Autodesk Inventor part; units mm, degrees
ref_plane "YZ Plane" through (0, 0, 0) normal (1, 0, 0) x (0, 1, 0)
ref_plane "XZ Plane" through (0, 0, 0) normal (0, 1, 0) x (-1, 0, 0)
ref_plane "XY Plane" through (0, 0, 0) normal (0, 0, 1) x (1, 0, 0)
sketch "Sketch1" plane through (0, 0, 0) normal (0, 0, 1) x (1, 0, 0)
  line L0 (0, 0) -> (140, 0)
  line L1 (140, 0) -> (140, 232.6)
  line L2 (140, 232.6) -> (90, 232.6)
  line L3 (90, 232.6) -> (90, 100)
  line L4 (90, 100) -> (50, 100)
  line L5 (50, 100) -> (50, 232.6)
  line L6 (50, 232.6) -> (0, 232.6)
  line L7 (0, 232.6) -> (0, 0)
  line L8 (30, 232.6) -> (30, 0) construction
  line L9 (70, 100) -> (70, 0) construction
  circle A0 centre (30, 192.6) radius 14 construction
  circle A1 centre (30, 152.6) radius 14 construction
  dimension "d3" = 40
  dimension "d6" = 28
  dimension "d7" = 40
  dimension "d8" = 40
  dimension "d9" = 132.6
  dimension "d10" = 100
  dimension "d36" = 20
  dimension "d37" = 50
extrude "Extrusion1" add sketch "Sketch1" along normal blind 3
ref_plane "Work Plane1" through (115, 0, 0) normal (1, 0, 0) x (0, 0, -1)
sketch "Sketch2" plane through (0, 0, 3) normal (0, 0, 1) x (1, 0, 0)
  line L0 (50, 232.6) -> (0, 232.6) construction
  line L1 (30, 232.6) -> (30, 50) construction
  line L2 (90, 100) -> (50, 100) construction
  line L3 (70, 100) -> (70, 0) construction
  line L4 (0, 0) -> (140, 0) construction
  circle A0 centre (30, 194.6) radius 14.25
  circle A1 centre (30, 134.6) radius 14.25
  circle A2 centre (30, 202.6) radius 4.6 construction
  circle A3 centre (110, 194.6) radius 14.25
  circle A4 centre (110, 134.6) radius 14.25
  line L5 (50, 100) -> (50, 232.6)
  dimension "d13" = 28.5
  dimension "d14" = 9.2
  dimension "d15" = 8
  dimension "d16" = 60
  dimension "d33" = 30
  dimension "d38" = 20
extrude "Extrusion2" cut sketch "Sketch2" against normal blind 10
sketch "Sketch3" plane through (0, 0, 3) normal (0, 0, 1) x (1, 0, 0)
  line L0 (5, 227.6) -> (45, 227.6)
  line L1 (45, 227.6) -> (45, 224.6)
  line L2 (45, 224.6) -> (5, 224.6)
  line L3 (5, 224.6) -> (5, 227.6)
  line L4 (53, 95) -> (87, 95)
  line L5 (87, 95) -> (87, 92)
  line L6 (87, 92) -> (53, 92)
  line L7 (53, 92) -> (53, 95)
  line L8 (5, 8) -> (135, 8)
  line L9 (135, 8) -> (135, 5)
  line L10 (135, 5) -> (5, 5)
  line L11 (5, 5) -> (5, 8)
  circle A0 centre (110, 194.6) radius 14.25
  circle A1 centre (30, 134.6) radius 14.25
  circle A2 centre (110, 134.6) radius 14.25
  circle A3 centre (30, 194.6) radius 14.25
  line L12 (50, 100) -> (50, 232.6)
  line L13 (50, 232.6) -> (0, 232.6)
  line L14 (0, 232.6) -> (0, 0)
  line L15 (0, 0) -> (140, 0)
  line L16 (140, 0) -> (140, 232.6)
  line L17 (140, 232.6) -> (90, 232.6)
  line L18 (90, 232.6) -> (90, 100)
  line L19 (90, 100) -> (50, 100)
  line L20 (90, 100) -> (50, 100) construction
  line L21 (70, 100) -> (70, 0) construction
  line L22 (0, 0) -> (140, 0) construction
  line L23 (135, 227.6) -> (95, 227.6)
  line L24 (95, 227.6) -> (95, 224.6)
  line L25 (95, 224.6) -> (135, 224.6)
  line L26 (135, 224.6) -> (135, 227.6)
  dimension "d20" = 5
  dimension "d21" = 5
  dimension "d22" = 5
  dimension "d23" = 3
  dimension "d24" = 5
  dimension "d25" = 3
  dimension "d26" = 3
  dimension "d27" = 3
  dimension "d28" = 5
  dimension "d29" = 3
  dimension "d30" = 5
extrude "Extrusion3" cut sketch "Sketch3" against normal blind 10 contours L0 L1 L2 L3 | L4 L5 L6 L7 | L8 L9 L10 L11 | L26 L25 L24 L23
ref_plane "Work Plane2" through (70, 0, 0) normal (1, 0, 0) x (0, 0, -1)
equation "\"d3\" = 0.5 * marshdistance"
equation "\"d9\" = sidewallL"
equation "\"d10\" = Uthick"
equation "\"d36\" = 0.5 * Utip"
equation "\"d16\" = marshmarshD"
equation "\"d33\" = marshedgeD"
equation "\"d38\" = 0.5 * Utip"
equation "\"thick\" = 0.5"
equation "\"lrlr\" = 19"
equation "\"lrmid\" = 19.9"
equation "\"lrdepth\" = 3.3"
equation "\"mlr\" = 16.6"
equation "\"mmid\" = 24.7"
equation "\"mdepth\" = 4.5"
equation "\"lrltotal\" = 126.6"
equation "\"mltotal\" = 126.6"
equation "\"lrbetween\" = 52.1"
equation "\"mbetween\" = 49.5"
equation "\"toler\" = 1"
equation "\"tight\" = 0.08"
equation "\"stuckw\" = 6"
equation "\"sidewallL\" = 132.6"
equation "\"heaterH\" = 117.3"
equation "\"Uthick\" = 100"
equation "\"marshmarshD\" = 60"
equation "\"marshedgeD\" = 30"
equation "\"stickL\" = 3.5"
equation "\"wireH\" = 25"
properties part number "Ushape_bottom"
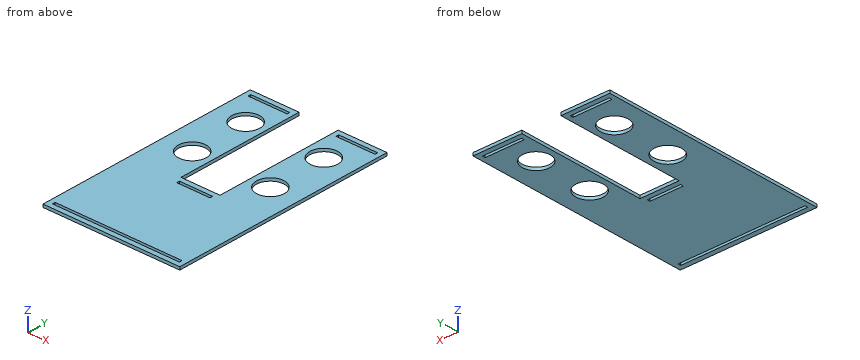
Verification items for the finished model (mm, model axes). Coordinates: 2 decimals unless noted, no trailing zeros. Write each loop counter-clockwise with the first axis right and the second up, starting at its lowest first coordinate (ties: lowest second). Pieces come first, ordered by that corner, then holes. Notation, with made-up numbers: (30.25, -28.5) -> (88.25, -28.5) arc R29 cw to (88.25, 6.5) -> close; hole circle Ø6 at (16.5, 45). An arc over 180 degrees is marked (long way). One line per item, written item: value. Start each with the question number.
Q1. Cross-section at B-B on y = 117. Enter the section's corners in (x, z).
Q2. Cross-section at D-D on z = 0.7. State how many separate pieces and enclosed holes the cut face has, and give its area (3 significant figures).
Q3. Thickness scan on L1, parallel to Y at x = 71, z = 0.3; L2, parallel to Y at x = 30, z = 2.1; L3, parallel to X at y = 186, z = 0.45. Record the ranges inside material, lowest first. Write a range as from..to.
Q4. Cross-section at A-A on x = 30. Enter the section's corners in (y, z), and give its area (3 significant figures).
Q5. Cross-section at C-C on y = 194.6. Enter the section's corners in (x, z), and give its area (3 significant figures).
Q6. Go/stop test with flat-tipped pins: P1, Ø17, axis at x = 30, y = 194.6, coming from the +Z side (3 decimals); P2, Ø1.5, axis at x = 63.5, z = 1.5, coming from the +Y side. Record where each tip stops, or that it passes through.
Checked values:
1. outline: (0, 0) -> (50, 0) -> (50, 3) -> (0, 3) -> close; (90, 0) -> (140, 0) -> (140, 3) -> (90, 3) -> close
2. separate pieces: 1
2. enclosed holes: 8
2. area: 24,000 mm²
3. L1: y = 0..5, 8..92, 95..100
3. L2: y = 0..5, 8..120.35, 148.85..180.35, 208.85..224.6, 227.6..232.6
3. L3: x = 0..18.64, 41.36..50, 90..98.64, 121.36..140
4. outline: (0, 0) -> (5, 0) -> (5, 3) -> (0, 3) -> close; (8, 0) -> (120.35, 0) -> (120.35, 3) -> (8, 3) -> close; (148.85, 0) -> (180.35, 0) -> (180.35, 3) -> (148.85, 3) -> close; (208.85, 0) -> (224.6, 0) -> (224.6, 3) -> (208.85, 3) -> close; (227.6, 0) -> (232.6, 0) -> (232.6, 3) -> (227.6, 3) -> close
4. area: 509 mm²
5. outline: (0, 0) -> (15.75, 0) -> (15.75, 3) -> (0, 3) -> close; (44.25, 0) -> (50, 0) -> (50, 3) -> (44.25, 3) -> close; (90, 0) -> (95.75, 0) -> (95.75, 3) -> (90, 3) -> close; (124.25, 0) -> (140, 0) -> (140, 3) -> (124.25, 3) -> close
5. area: 129 mm²
6. P1: passes through
6. P2: stops at y = 100
